For this review, take the finished solid that the model builds, in its own axes (mm). Face numbers are marked on the shaded views. A direction names the side the tool comes from. Give positions to 0.01 mm unless a question says otherwise; leave off trailing zeros. Order: outer loops, then holes, each group sorted by start corner. A loop starts at its lowest first (then second) coordinate and runs counter-clockwise, first axis right, second up.
Item 1: Consider section A-A (y = 0). Give the boundary of the cut face in (x, z) (3 decimals), plus the area to 3 significant figures.
Item 2: For probe 1 along Y at (x, z) = (-82.5, 20) (3 decimals); probe 2 along Y at (x, z) = (1.5, 14.25) (3 decimals); probe 3 along X at (y, z) = (-5, 21), list the stretches that pass through material, from the lowest coordinate up.
Item 3: The part is to be moulded in two halves that separate along X. For the marked faces 3, 4 and 5, say which applies: released by +X, released by -X, zero draft, split by the parting line, or undercut.
Item 4: Machinability: for the marked faces 1 and 2, which of the approach directions +Z, -Z, +X, -X, +Y, -Y give a long, thin tool a straight path to every point of the face, cutting with its end or side? Answer none if there is none.
Item 5: For P1, Ø5, axis at x = -31, y = -50, coming from the +Z side (3 decimals); P2, Ø2.5, axis at x = 98.5, y = 1, coming from the -Z side; P3, Ø9.5, axis at x = 46, y = -5.5, coming from the +Z side (3 decimals), all flat-tipped, find the tip position at first contact; note any pin that passes through.
Item 6: Consider section B-B (x = -30.5). Give the boundary of the cut face in (y, z) (3 decimals), plus the area to 3 significant figures.
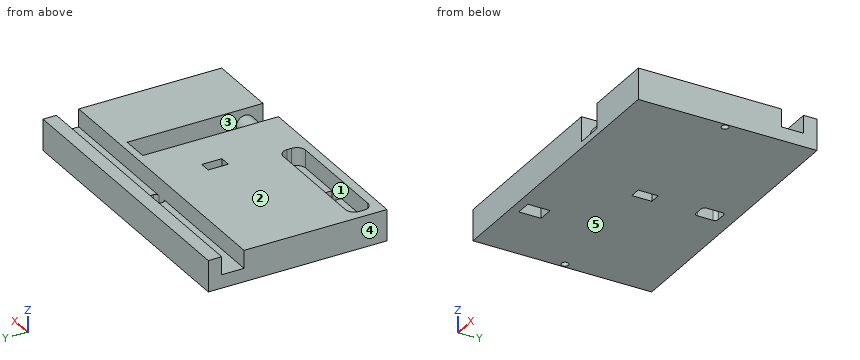
```python
from build123d import *

# Parameters (mm, degrees)
F0_W     = 7.9375
F0_H     = 14.2875
F1_DEPTH = 9.525
F2_DEPTH = 22.225
F3_R     = 6.35
F4_DEPTH = 80.518
F0_W_2   = 19.0754
F0_H_2   = 96.52
F5_DEPTH = 4.445
F6_R     = 2.54
F7_DEPTH = 12.7


with BuildPart() as f1:
    # F0 (on Top) → F1 (new body)
    with BuildSketch(Plane.XY):
        Polygon((-101.6, 38.1), (-101.6, -63.5), (31.7246, -63.5), (31.7246, 33.02), (50.8, 33.02), (50.8, -63.5), (101.6, -63.5), (101.6, 38.1), (3.0768760622, 38.1), (-3.0768760622, 38.1), align=None)
        with BuildLine():
            Line((-56.3626, -57.15), (-88.9, -57.15))
            ThreePointArc((-88.9, -57.15), (-93.3901280605, -55.2901280605), (-95.25, -50.8))
            Line((-95.25, -50.8), (-95.25, -47.625))
            ThreePointArc((-95.25, -47.625), (-93.3901280605, -43.1348719395), (-88.9, -41.275))
            Line((-88.9, -41.275), (-56.3626, -41.275))
            Line((-56.3626, -41.275), (-45.2374, -41.275))
            Line((-45.2374, -41.275), (-12.7, -41.275))
            ThreePointArc((-12.7, -41.275), (-8.2098719395, -43.1348719395), (-6.35, -47.625))
            Line((-6.35, -47.625), (-6.35, -50.8))
            ThreePointArc((-6.35, -50.8), (-8.2098719395, -55.2901280605), (-12.7, -57.15))
            Line((-12.7, -57.15), (-45.2374, -57.15))
            Line((-45.2374, -57.15), (-56.3626, -57.15))
        make_face(mode=Mode.SUBTRACT)
        Rectangle(F0_W, F0_H, mode=Mode.SUBTRACT)
        Polygon((-101.6, 63.5), (-101.6, 53.975), (-3.0768760622, 53.975), (3.0768760622, 53.975), (101.6, 53.975), (101.6, 63.5), align=None)
        with BuildLine():
            Line((-101.6, 53.975), (-101.6, 38.1))
            Line((-101.6, 38.1), (-3.0768760622, 38.1))
            ThreePointArc((-3.0768760622, 38.1), (-4.8300581867, 38.8261918133), (-5.55625, 40.5793739378))
            Line((-5.55625, 40.5793739378), (-5.55625, 51.4956260622))
            ThreePointArc((-5.55625, 51.4956260622), (-4.8300581867, 53.2488081867), (-3.0768760622, 53.975))
            Line((-3.0768760622, 53.975), (-101.6, 53.975))
        make_face()
        with BuildLine():
            ThreePointArc((5.55625, 40.5793739378), (4.8300581867, 38.8261918133), (3.0768760622, 38.1))
            Line((3.0768760622, 38.1), (101.6, 38.1))
            Line((101.6, 38.1), (101.6, 53.975))
            Line((101.6, 53.975), (3.0768760622, 53.975))
            ThreePointArc((3.0768760622, 53.975), (4.8300581867, 53.2488081867), (5.55625, 51.4956260622))
            Line((5.55625, 51.4956260622), (5.55625, 40.5793739378))
        make_face()
        with BuildLine():
            ThreePointArc((-95.25, -50.8), (-93.3901280605, -55.2901280605), (-88.9, -57.15))
            Line((-88.9, -57.15), (-56.3626, -57.15))
            Line((-56.3626, -57.15), (-56.3626, -41.275))
            Line((-56.3626, -41.275), (-88.9, -41.275))
            ThreePointArc((-88.9, -41.275), (-93.3901280605, -43.1348719395), (-95.25, -47.625))
            Line((-95.25, -47.625), (-95.25, -50.8))
        make_face()
        with BuildLine():
            Line((-45.2374, -41.275), (-45.2374, -57.15))
            Line((-45.2374, -57.15), (-12.7, -57.15))
            ThreePointArc((-12.7, -57.15), (-8.2098719395, -55.2901280605), (-6.35, -50.8))
            Line((-6.35, -50.8), (-6.35, -47.625))
            ThreePointArc((-6.35, -47.625), (-8.2098719395, -43.1348719395), (-12.7, -41.275))
            Line((-12.7, -41.275), (-45.2374, -41.275))
        make_face()
    extrude(amount=F1_DEPTH)

    # F0 (on Top) → F2 (join)
    with BuildSketch(Plane.XY):
        Polygon((-101.6, 63.5), (-101.6, 53.975), (-3.0768760622, 53.975), (3.0768760622, 53.975), (101.6, 53.975), (101.6, 63.5), align=None)
        Polygon((-101.6, 38.1), (-101.6, -63.5), (31.7246, -63.5), (31.7246, 33.02), (50.8, 33.02), (50.8, -63.5), (101.6, -63.5), (101.6, 38.1), (3.0768760622, 38.1), (-3.0768760622, 38.1), align=None)
        with BuildLine():
            Line((-56.3626, -57.15), (-88.9, -57.15))
            ThreePointArc((-88.9, -57.15), (-93.3901280605, -55.2901280605), (-95.25, -50.8))
            Line((-95.25, -50.8), (-95.25, -47.625))
            ThreePointArc((-95.25, -47.625), (-93.3901280605, -43.1348719395), (-88.9, -41.275))
            Line((-88.9, -41.275), (-56.3626, -41.275))
            Line((-56.3626, -41.275), (-45.2374, -41.275))
            Line((-45.2374, -41.275), (-12.7, -41.275))
            ThreePointArc((-12.7, -41.275), (-8.2098719395, -43.1348719395), (-6.35, -47.625))
            Line((-6.35, -47.625), (-6.35, -50.8))
            ThreePointArc((-6.35, -50.8), (-8.2098719395, -55.2901280605), (-12.7, -57.15))
            Line((-12.7, -57.15), (-45.2374, -57.15))
            Line((-45.2374, -57.15), (-56.3626, -57.15))
        make_face(mode=Mode.SUBTRACT)
        Rectangle(F0_W, F0_H, mode=Mode.SUBTRACT)
    extrude(amount=F2_DEPTH)

    # F3 (on face) → F4 (join)
    with BuildSketch(Plane.YZ.offset(101.6)):
        with Locations((-50.8, 11.1125)):
            Circle(F3_R)
    extrude(amount=-F4_DEPTH)

    # F0 (on Top) → F5 (join)
    with BuildSketch(Plane.XY):
        with Locations((41.2623, -15.24)):
            Rectangle(F0_W_2, F0_H_2)
    extrude(amount=F5_DEPTH)

    # F6 (on face) → F7 (cut)
    with BuildSketch(Plane.XY):
        with Locations((-98.425, 0)):
            Circle(F6_R)
        with Locations((98.425, 0)):
            Circle(F6_R)
    extrude(amount=F7_DEPTH, mode=Mode.SUBTRACT)


solid = f1.part
```
Resolved:
1. outline: (-101.6, 0) - (-100.965, 0) - (-100.965, 12.7) - (-95.885, 12.7) - (-95.885, 0) - (-3.969, 0) - (-3.969, 22.225) - (-101.6, 22.225) - close; (3.969, 0) - (95.885, 0) - (95.885, 12.7) - (100.965, 12.7) - (100.965, 0) - (101.6, 0) - (101.6, 22.225) - (50.8, 22.225) - (50.8, 4.445) - (31.725, 4.445) - (31.725, 22.225) - (3.969, 22.225) - close
1. area: 3,870 mm2
2. probe 1: y = -63.5 to -57.15, -41.275 to 38.1, 53.975 to 63.5
2. probe 2: y = -63.5 to -7.144, 7.144 to 38.1, 53.975 to 63.5
2. probe 3: x = -101.6 to -3.97, 3.97 to 31.72, 50.8 to 101.6
3. face 3: undercut
3. face 4: released by -X
3. face 5: zero draft
4. face 1: +Z
4. face 2: +Z, +X, -X, +Y, -Y
5. P1: stops at z = 9.525
5. P2: stops at z = 12.7
5. P3: stops at z = 4.445
6. outline: (-63.5, 0) - (63.5, 0) - (63.5, 22.225) - (53.975, 22.225) - (53.975, 9.525) - (38.1, 9.525) - (38.1, 22.225) - (-41.275, 22.225) - (-41.275, 9.525) - (-57.15, 9.525) - (-57.15, 22.225) - (-63.5, 22.225) - close
6. area: 2,420 mm2
